from build123d import *

# Parameters (mm, degrees)
SKETCH1_R           = 1.925
BOSS_EXTRUDE1_DEPTH = 3.175


with BuildPart() as part:
    # Sketch1 → Boss-Extrude1 (new body)
    with BuildSketch(Plane.XY):
        with BuildLine():
            Line((1.75, 90.718911087), (17.75, 90.718911087))
            Line((17.75, 90.718911087), (17.75, 83.718911087))
            Line((17.75, 83.718911087), (11.75, 83.718911087))
            ThreePointArc((11.75, 83.718911087), (4.678932188, 80.789978899), (1.75, 73.718911087))
            Line((1.75, 73.718911087), (1.75, 5.986860279))
            ThreePointArc((1.75, 5.986860279), (1.784074174, 5.728041234), (1.883974596, 5.486860279))
            Line((1.883974596, 5.486860279), (6.062177826, -1.75))
            ThreePointArc((6.062177826, -1.75), (4.744524835, -4.363775134), (2.873226135, -2.112937283))
            ThreePointArc((2.873226135, -2.112937283), (2.91057922, -1.707249179), (2.783018833, -1.320330017))
            Line((2.783018833, -1.320330017), (0.866025404, 2))
            ThreePointArc((0.866025404, 2), (0, 2.5), (-0.866025404, 2))
            Line((-0.866025404, 2), (-2.783018833, -1.320330017))
            ThreePointArc((-2.783018833, -1.320330017), (-2.91057922, -1.707249179), (-2.873226135, -2.112937283))
            ThreePointArc((-2.873226135, -2.112937283), (-4.744524835, -4.363775134), (-6.062177826, -1.75))
            Line((-6.062177826, -1.75), (-1.883974596, 5.486860279))
            ThreePointArc((-1.883974596, 5.486860279), (-1.784074174, 5.728041234), (-1.75, 5.986860279))
            Line((-1.75, 5.986860279), (-1.75, 73.718911087))
            ThreePointArc((-1.75, 73.718911087), (-4.678932188, 80.789978899), (-11.75, 83.718911087))
            Line((-11.75, 83.718911087), (-17.75, 83.718911087))
            Line((-17.75, 83.718911087), (-17.75, 90.718911087))
            Line((-17.75, 90.718911087), (-1.75, 90.718911087))
            Line((-1.75, 90.718911087), (1.75, 90.718911087))
        make_face()
        with Locations((-13.75, 87.218911087)):
            Circle(SKETCH1_R, mode=Mode.SUBTRACT)
        with Locations((13.75, 87.218911087)):
            Circle(SKETCH1_R, mode=Mode.SUBTRACT)
    extrude(amount=BOSS_EXTRUDE1_DEPTH)


solid = part.part
The listing builds one solid part. Answer for the finished solid, in the listing's coordinates (mm). A direction names the side the tool comes from. Coordinates: 2 decimals unless noted, no trailing zeros. Loops run counter-clockwise (first coordinate to the right, second up) from the corner with the lowest first, then second, coordinate; pieces in that order, holes last. Notation, with made-up numbers: (35.25, 47) -> (68.25, 47) arc R21 ccw to (68.25, 59) -> close; hole circle Ø2 at (40.5, 54). An arc over 180 degrees is marked (long way). Write item = value, one per line. Start each with the question number.
1) A cutting plane is placed at B-B (y = 35). Give the vertices of the cut face in (x, z) (3 decimals).
2) A cutting plane is placed at A-A (x = 13.75). Give the vertices of the cut face in (y, z) (3 decimals), then the cut area to 3 significant figures.
3) A cutting plane is placed at C-C (z = 0.9). Give the vertices of the cut face in (x, y) (3 decimals), then the cut area to 3 significant figures.
4) The mould has two halves that part along Y. Classify faces 5 (the face through (-4.7, -4.37, 1.57)), 6 (the face through (0, 90.719, 2)), 7 (the face through (17.75, 87, 2)): released by +Y, released by -Y, zero draft, split by the parting line, or undercut.
5) A tool of negligible diameter and unlimited length cuts with its end or side. For faces 1 (the face through (-1.811, 0.363, 1.565)), 2 (the face through (1.75, 40, 2)), 3 (the face through (-15, 83.719, 2)), 4 (the face through (15, 83.719, 2)), from which of +Z, -Z, +X, -X, +Y, -Y can it reach the whole face along a straight path? Write none if from no direction.
6) Given pin 1 Ø1 at (x, z) = (-13.5, 1) entering from -Y; pin 2 Ø1.6 at (y, z) = (49, 1.5) entering from -X, each flat-ended and moving along its own axis, determine where each tip first touches the part or whether it passes through.
7) Straight lines are drawn through the part: line 1 (Y direction, x = 14, z = 0.1); line 2 (X direction, y = 28.5, z = 2.15); line 3 (X direction, y = 0.5, z = 0.8). For each, find the intervals that lie inside material, in ascending order. Write a range as from..to.
8) A cutting plane is placed at D-D (x = -13). Give the vertices of the cut face in (y, z) (3 decimals).
Responses:
q1.outline = (-1.75, 0) -> (1.75, 0) -> (1.75, 3.175) -> (-1.75, 3.175) -> close
q2.outline = (83.719, 0) -> (85.294, 0) -> (85.294, 3.175) -> (83.719, 3.175) -> close; (89.144, 0) -> (90.719, 0) -> (90.719, 3.175) -> (89.144, 3.175) -> close
q2.area = 10.0 mm²
q3.outline = (-17.75, 83.719) -> (-11.75, 83.719) arc R10 cw to (-1.75, 73.719) -> (-1.75, 5.987) arc R1 cw to (-1.884, 5.487) -> (-6.062, -1.75) arc R1.75 ccw (long way) to (-2.873, -2.113) arc R1 cw to (-2.783, -1.32) -> (-0.866, 2) arc R1 cw to (0.866, 2) -> (2.783, -1.32) arc R1 cw to (2.873, -2.113) arc R1.75 ccw (long way) to (6.062, -1.75) -> (1.884, 5.487) arc R1 cw to (1.75, 5.987) -> (1.75, 73.719) arc R10 cw to (11.75, 83.719) -> (17.75, 83.719) -> (17.75, 90.719) -> (-17.75, 90.719) -> close; hole circle Ø3.85 at (-13.75, 87.219); hole circle Ø3.85 at (13.75, 87.219)
q3.area = 600 mm²
q4.face_5 = undercut
q4.face_6 = released by +Y
q4.face_7 = zero draft
q5.face_1 = +Z, -Z, -Y
q5.face_2 = +Z, -Z, +X
q5.face_3 = +Z, -Z, -X, -Y
q5.face_4 = +Z, -Z, +X, -Y
q6.pin_1 = 83.72
q6.pin_2 = -1.75
q7.line_1 = 83.72..85.31, 89.13..90.72
q7.line_2 = -1.75..1.75
q7.line_3 = -4.76..-1.73, 1.73..4.76
q8.outline = (83.719, 0) -> (85.446, 0) -> (85.446, 3.175) -> (83.719, 3.175) -> close; (88.992, 0) -> (90.719, 0) -> (90.719, 3.175) -> (88.992, 3.175) -> close
